Verification items for this drawing (mm, ordinates from the low corner). Give positions to 0.01 mm unless a question says otherwise; leave off trailing zeros. Write each loop counter-clockwise with the first axis right and the second up, starting at its lowest first coordinate (ties: lowest second). Pieces come first, ordered by that corner, then holes. Notation, with made-up numbers: (46.5, 19) -> (94.5, 19) arc R20 ccw to (94.5, 58) -> close; hole circle Ø6 at (-31.75, 78). An arc over 180 degrees is marked (long way). One line per item, written item: value.
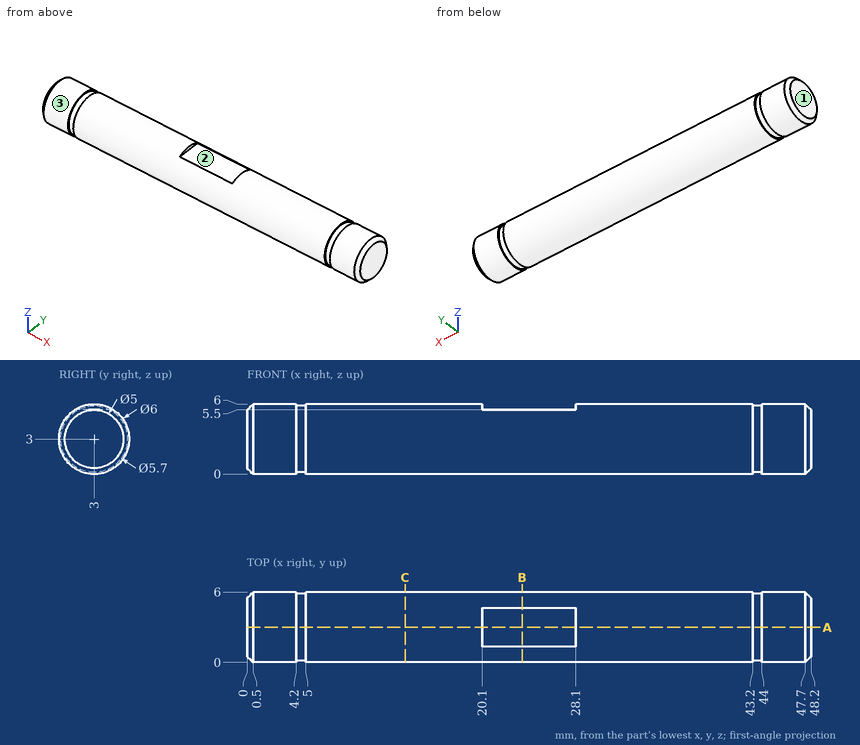
1) Scan lines: probe 1 along Y at (x, z) = (25, 3.25); probe 2 along Y at (x, z) = (29, 1.25); probe 3 along Z at (x, y) = (31.5, 2.65). Record each from-to range of solid material in increasing order.
Verdict:
probe 1: 0.01 to 5.99
probe 2: 0.56 to 5.44
probe 3: 0.02 to 5.98
2) Sectioned sample at C-C on x = 13.5. Record the cut outline in (y, z), plus the area to 3 significant figures.
Verdict:
outline: circle Ø6 at (3, 3)
area: 28.3 mm^2
3) Depth check by flat-ended pin: pin 1 Ø3.5 at (x, y) = (22, 3.5) entering from +Z; pin 2 Ø1.5 at (x, z) = (29, 1) entering from +Y. Enter the tip coordinate at first touch or a pass-through.
Verdict:
pin 1: z = 5.5
pin 2: y = 5.73
4) Mould release check, pull along X, two halves, no side actions. Record for the marked faces 1, 2 and 3: released by +X, released by -X, zero draft, split by the parting line, or undercut.
Verdict:
face 1: released by -X
face 2: undercut
face 3: zero draft
5) Sectioned sample at A-A on y = 3. Record the cut outline in (x, z).
Verdict:
outline: (0, 0.5) -> (0.5, 0) -> (4.2, 0) -> (4.2, 0.15) -> (5, 0.15) -> (5, 0) -> (43.2, 0) -> (43.2, 0.15) -> (44, 0.15) -> (44, 0) -> (47.7, 0) -> (48.2, 0.5) -> (48.2, 5.5) -> (47.7, 6) -> (44, 6) -> (44, 5.85) -> (43.2, 5.85) -> (43.2, 6) -> (28.1, 6) -> (28.1, 5.5) -> (20.1, 5.5) -> (20.1, 6) -> (5, 6) -> (5, 5.85) -> (4.2, 5.85) -> (4.2, 6) -> (0.5, 6) -> (0, 5.5) -> close
6) Sectioned sample at B-B on x = 23.5. Record the cut outline in (y, z), plus the area to 3 significant figures.
Verdict:
outline: (1.34, 5.5) arc R3 ccw (long way) to (4.66, 5.5) -> close
area: 27.1 mm^2
